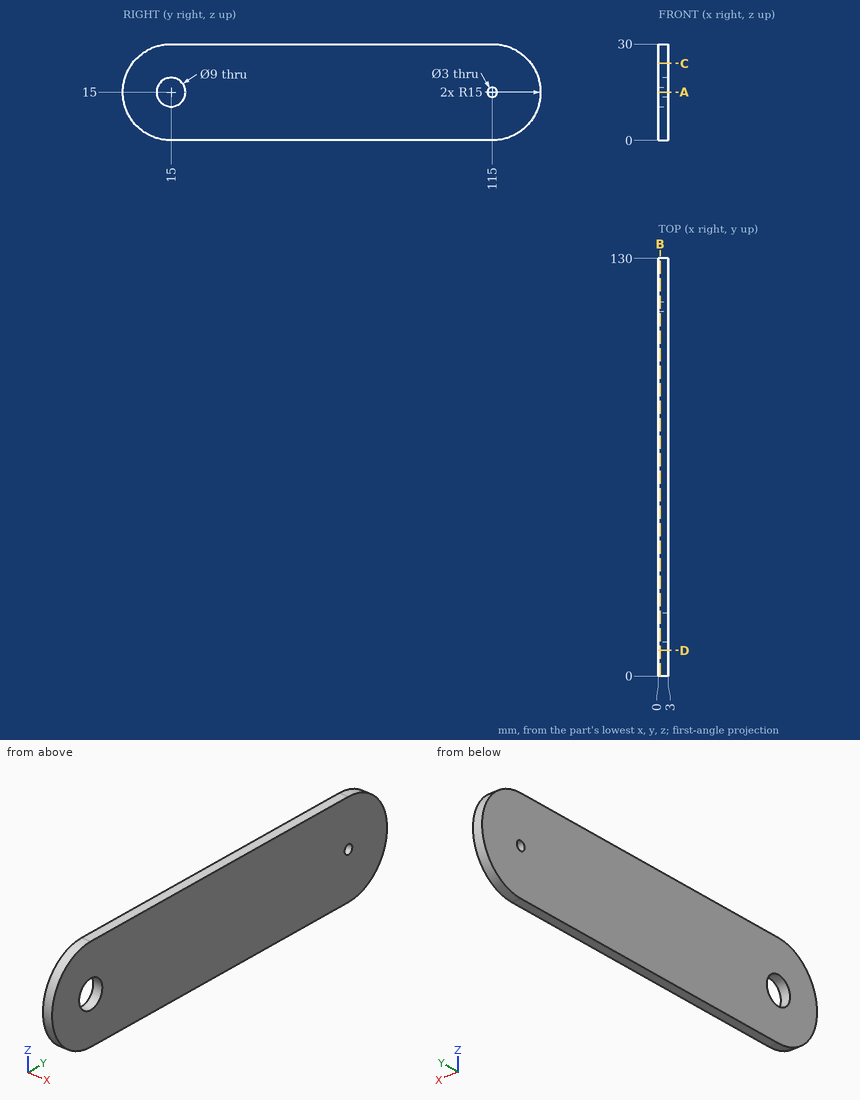
Geometry: see drawing. Coordinates: mm, zero at the bounding-box minimum. Give positions to 0.01 mm unless a question says otherwise; leave off trailing zeros. Write each loop counter-clockwise with the first axis right and the second up, starting at its lowest first coordinate (ties: lowest second). Pieces come first, ordered by that corner, then holes. Notation, with made-up numbers: M 52.5,75.5 L 71.5,75.5 A12 cw 71.5,79.5 Z; hole C 88.5,6.25 d11. An arc over 180 degrees is marked long. Answer as a JSON object with one key per item and string values.
Q1. Contact query for flat-ended pins moving along their axis: P1, Ø8, axis at y = 15, z = 15, coming from the +X side; P2, Ø1.5, axis at x = 0.5, z = 17.5, coming from the +Y side. Output: stop coordinate, or through.
Geometry check:
{"P1": "passes through", "P2": "stops at y = 129.9"}
Q2. Cut plane D-D, the plane y = 8. Return the cut outline in (x, z), then the cut area to 3 significant figures.
Geometry check:
{"outline": "M 0,1.73 L 3,1.73 L 3,28.27 L 0,28.27 Z", "area": "79.6 mm^2"}
Q3. Cut plane C-C, the plane z = 24. Return the cut outline in (x, y).
Geometry check:
{"outline": "M 0,3 L 3,3 L 3,127 L 0,127 Z"}
Q4. Cut plane B-B, the plane x = 0.5. Return the cut outline in (y, z).
Geometry check:
{"outline": "M 15,0 L 115,0 A15 ccw 115,30 L 15,30 A15 ccw Z; hole C 15,15 d9; hole C 115,15 d3"}
Q5. Cut plane A-A, the plane z = 15. Return the cut outline in (x, y).
Geometry check:
{"outline": "M 0,0 L 3,0 L 3,10.5 L 0,10.5 Z; M 0,19.5 L 3,19.5 L 3,113.5 L 0,113.5 Z; M 0,116.5 L 3,116.5 L 3,130 L 0,130 Z"}
Q6. Ray query, line 1 along Y through (x, z) = (2.2, 15); line 2 along Z through (x, y) = (1.7, 115); line 3 along Y through (x, z) = (0.9, 11). Return the intervals inside material, ascending.
Geometry check:
{"line 1": "y = 0 to 10.5, 19.5 to 113.5, 116.5 to 130", "line 2": "z = 0 to 13.5, 16.5 to 30", "line 3": "y = 0.54 to 12.94, 17.06 to 129.46"}
